The listing builds one solid part. Answer for the finished solid, in the listing's coordinates (mm). Round coordinates to 2 decimals unless told otherwise and drop trailing zeros. Order: outer loops, then holes, each group sorted by start corner. A loop starts at its lowest first (then second) coordinate and runs counter-clockwise, first axis right, second up. Notation, with made-up numbers: (48, -19) - (74, -19) arc R24 ccw to (74, 9) - close; hole circle Ø1 at (8, -4). An arc over 180 degrees is marked (long way). One line per item, written item: value. Start each with the question number.
1. Section A-A, the plane y = 82.5 is taken. Give the vertices of the cut face in (x, z).
2. Section B-B, the plane z = -2 is taken. Give the vertices of the cut face in (x, y).
3. Straight lines are drawn through the part: line 1 (Y direction, x = 0.5, z = -0.35); line 2 (Y direction, x = -183, z = -1.8); line 3 (X direction, y = 86.5, z = -1.45). For each, find the intervals that lie inside material, in ascending order.
4. Section D-D, the plane x = 0 is taken. Give the vertices of the cut face in (y, z).
5. Section C-C, the plane y = -36 is taken. Give the vertices of the cut face in (x, z).
6. A flat-ended cylindrical pin translates along its axis: P1, Ø1.5, axis at x = 199.5, z = -0.5, coming from the +Y side. Find the tip coordinate at first contact, or state that the pin passes through.
Autodesk Inventor part; units mm, degrees
ref_plane "YZ Plane" through (0, 0, 0) normal (1, 0, 0) x (0, 1, 0)
ref_plane "XZ Plane" through (0, 0, 0) normal (0, 1, 0) x (-1, 0, 0)
ref_plane "XY Plane" through (0, 0, 0) normal (0, 0, 1) x (1, 0, 0)
sketch "Sketch1" plane through (0, 0, 0) normal (0, 0, 1) x (1, 0, 0)
  arc A0 (100, 0) -> (-100, 0) centre (0, 0) ccw
  arc A1 (267.9086, -135) -> (-267.9086, -135) centre (0, 0) ccw
  line L0 (-100, 0) -> (-100, -135)
  line L1 (-100, -135) -> (-267.9086, -135)
  line L2 (100, 0) -> (100, -135)
  line L3 (100, -135) -> (267.9086, -135)
  dimension "d0" = 200
  dimension "d2" = 600
  dimension "d3" = 135
extrude "Extrusion1" add sketch "Sketch1" against normal blind 3
sketch "Sketch2" plane through (0, 0, 0) normal (0, 0, 1) x (1, 0, 0)
  arc A0 (100, 0) -> (-100, 0) centre (0, 0) ccw
  line L0 (100, 0) -> (100, -135)
  line L1 (100, -135) -> (267.9086, -135)
  arc A1 (267.9086, -135) -> (-267.9086, -135) centre (0, 0) ccw
  line L2 (-267.9086, -135) -> (-100, -135)
  line L3 (-100, -135) -> (-100, 0)
  line L4 (-101.709, 282.2327) -> (100, 282.2327)
  line L5 (100, 282.2327) -> (100, 100)
  line L6 (100, 100) -> (-101.709, 100)
  line L7 (-101.709, 100) -> (-101.709, 282.2327)
properties part number "bed"
Answer list:
1. outline: (-288.43, -3) - (-56.51, -3) - (-56.51, 0) - (-288.43, 0) - close; (56.51, -3) - (288.43, -3) - (288.43, 0) - (56.51, 0) - close
2. outline: (-267.91, -135) - (-100, -135) - (-100, 0) arc R100 cw to (100, 0) - (100, -135) - (267.91, -135) arc R300 ccw (long way) to start
3. line 1: y = 100 to 300
3. line 2: y = -135 to 237.72
3. line 3: x = -287.26 to -50.18, 50.18 to 287.26
4. outline: (100, -3) - (300, -3) - (300, 0) - (100, 0) - close
5. outline: (-297.83, -3) - (-100, -3) - (-100, 0) - (-297.83, 0) - close; (100, -3) - (297.83, -3) - (297.83, 0) - (100, 0) - close
6. P1: stops at y = 224.72
